```python
from build123d import *

# Parameters (mm, degrees)
SKETCH1_R                                       = 2.5
BOSS_EXTRUDE1_DEPTH                             = 35
SKETCH2_W                                       = 19.147849822
SKETCH2_H                                       = 14
CUT_EXTRUDE1_DEPTH                              = 11.980294351
CUT_EXTRUDE1_DEPTH_BACK                         = 1
CSK_FOR_M5_FLAT_HEAD_MACHINE_SCREW1_D           = 5.5
CSK_FOR_M5_FLAT_HEAD_MACHINE_SCREW1_DEPTH       = 13.347633298
CSK_FOR_M5_FLAT_HEAD_MACHINE_SCREW1_CSINK_D     = 10.4
CSK_FOR_M5_FLAT_HEAD_MACHINE_SCREW1_CSINK_ANGLE = 90
CSK_FOR_M5_FLAT_HEAD_MACHINE_SCREW1_TIP         = 1.652366702
CUT_EXTRUDE2_START                              = -14
SKETCH6_R                                       = 5.25
CUT_EXTRUDE2_DEPTH                              = 14
CUT_EXTRUDE3_START                              = -42
SKETCH6_2_R                                     = 5.25
CUT_EXTRUDE3_DEPTH                              = 14


with BuildPart() as part:
    # Sketch1 → Boss-Extrude1 (new body, symmetric)
    with BuildSketch(Plane(origin=(0, 0, 0), x_dir=(1, 0, 0), z_dir=(0, 1, 0))):
        with BuildLine():
            Line((0, 0), (28, 0))
            Line((28, 0), (28, -1.5))
            ThreePointArc((28, -1.5), (34.920820135, -7.683011565), (25.645751311, -8))
            Line((25.645751311, -8), (2.645751311, -8))
            Line((2.645751311, -8), (0, -5))
            Line((0, -5), (0, 0))
        make_face()
        with Locations((30.219676222, -5.980294351)):
            Circle(SKETCH1_R, mode=Mode.SUBTRACT)
    extrude(amount=BOSS_EXTRUDE1_DEPTH, both=True)

    # Sketch2 → Cut-Extrude1 (cut, two sides)
    with BuildSketch(Plane.XY) as cut_extrude1_sk:
        with Locations((35.219676222, 14)):
            Rectangle(SKETCH2_W, SKETCH2_H)
        with Locations((35.219676222, -14)):
            Rectangle(SKETCH2_W, SKETCH2_H)
    extrude(amount=CUT_EXTRUDE1_DEPTH, mode=Mode.SUBTRACT)
    extrude(cut_extrude1_sk.sketch, amount=-CUT_EXTRUDE1_DEPTH_BACK, mode=Mode.SUBTRACT)

    # CSK for M5 Flat Head Machine Screw1
    with Locations(Plane.XY.offset(8)):
        with Locations((12.432713767, 18), (12.432713767, -18)):
            CounterSinkHole(CSK_FOR_M5_FLAT_HEAD_MACHINE_SCREW1_D / 2, CSK_FOR_M5_FLAT_HEAD_MACHINE_SCREW1_CSINK_D / 2, depth=CSK_FOR_M5_FLAT_HEAD_MACHINE_SCREW1_DEPTH, counter_sink_angle=CSK_FOR_M5_FLAT_HEAD_MACHINE_SCREW1_CSINK_ANGLE)
            with Locations((0, 0, -(CSK_FOR_M5_FLAT_HEAD_MACHINE_SCREW1_DEPTH + CSK_FOR_M5_FLAT_HEAD_MACHINE_SCREW1_TIP / 2))):  # 118° drill point
                Cone(0, CSK_FOR_M5_FLAT_HEAD_MACHINE_SCREW1_D / 2, CSK_FOR_M5_FLAT_HEAD_MACHINE_SCREW1_TIP, mode=Mode.SUBTRACT)

    # Sketch6 → Cut-Extrude2 (cut)
    with BuildSketch(Plane(origin=(0, 35, 0), x_dir=(1, 0, 0), z_dir=(0, 1, 0)).offset(CUT_EXTRUDE2_START)):
        with Locations((30.219676222, -5.980294351)):
            Circle(SKETCH6_R)
    extrude(amount=-CUT_EXTRUDE2_DEPTH, mode=Mode.SUBTRACT)

    # Sketch6<2> → Cut-Extrude3 (cut)
    with BuildSketch(Plane(origin=(0, 35, 0), x_dir=(1, 0, 0), z_dir=(0, 1, 0)).offset(CUT_EXTRUDE3_START)):
        with Locations((30.219676222, -5.980294351)):
            Circle(SKETCH6_2_R)
    extrude(amount=-CUT_EXTRUDE3_DEPTH, mode=Mode.SUBTRACT)


solid = part.part
```
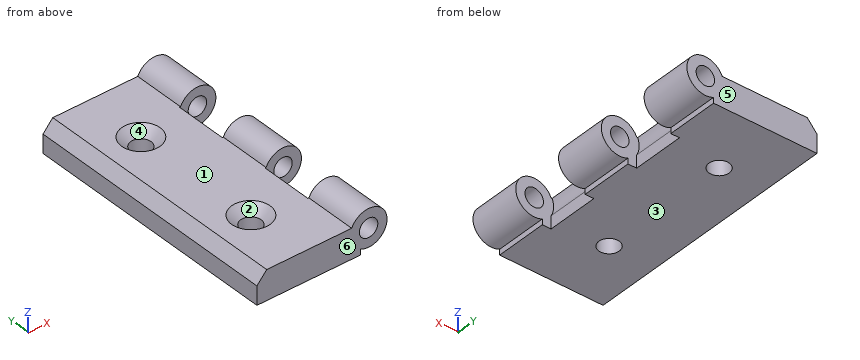
Design review of the part built by this model. Coordinates are the model's own, in mm. Face numbers are marked on the shaded views. A direction names the side the tool comes from. Round coordinates to 2 decimals unless told otherwise and drop trailing zeros. Write each loop counter-clockwise with the first axis right and the second up, starting at its lowest first coordinate (ties: lowest second). Pieces come first, ordered by that corner, then holes.
Item 1: We need section B-B on z = 2.25. Write out the cut boundary in (x, y).
Item 2: We need section D-D on x = 14.5. State how many separate pieces and enclosed holes the cut face has, and give its area (3 significant figures).
Item 3: The part is to be moulded in two halves that separate along Y. For the marked faces 3, 4, 5 and 6, say which applies: +Y half, -Y half, draft (parallel to the pull), parting line (faces both ways), or undercut.
Item 4: Clearance check with flat-ended pins moving along their axes: pin 1 Ø1 at (x, y) = (18, 22) entering from +Z; pin 2 Ø0.8 at (y, z) = (29.5, 0.5) entering from +X; pin 3 Ø1.5 at (y, z) = (-9.5, 6.5) entering from +X. State where each tip first meets the part, or that it passes through.
Item 5: We need section C-C on x = 33.5. Write out the cut boundary in (y, z).
Item 6: For probe 1 along Y at (x, z) = (12.5, 2.5); probe 2 along Y at (x, z) = (32, 8.75); probe 3 along X at (y, z) = (-2, 6.5), list the stretches that pass through material, from the lowest coordinate up.
Item 7: We need section A-A on y = -18. Write out the cut boundary in (x, z).
Item 8: For the marked faces 1 and 2, list the 3-axis set-ups (+Z, -Z, +X, -X, +Y, -Y) from which the entire face can be reached by the end or side of a thin tool; tool diameter is ignored.
Returned:
1. outline: (0, -35) - (33.55, -35) - (33.55, -21) - (25.65, -21) - (25.65, -7) - (33.55, -7) - (33.55, 7) - (25.65, 7) - (25.65, 21) - (33.55, 21) - (33.55, 35) - (0, 35) - close; hole circle Ø5.5 at (12.43, -18); hole circle Ø5.5 at (12.43, 18)
2. separate pieces: 3
2. enclosed holes: 0
2. area: 487 mm2
3. face 3: draft
3. face 4: undercut
3. face 5: +Y half
3. face 6: -Y half
4. pin 1: stops at z = 8
4. pin 2: stops at x = 28
4. pin 3: stops at x = 25.13
5. outline: (-35, 2.21) - (-21, 2.21) - (-21, 9.75) - (-35, 9.75) - close; (-7, 2.21) - (7, 2.21) - (7, 9.75) - (-7, 9.75) - close; (21, 2.21) - (35, 2.21) - (35, 9.75) - (21, 9.75) - close
6. probe 1: y = -35 to -20.75, -15.25 to 15.25, 20.75 to 35
6. probe 2: y = -35 to -21, -7 to 7, 21 to 35
6. probe 3: x = 1.32 to 27.77, 32.67 to 35.19
7. outline: (0, 0) - (9.68, 0) - (9.68, 5.55) - (7.23, 8) - (2.65, 8) - (0, 5) - close; (15.18, 0) - (25.65, 0) - (25.65, 3.4) arc R5.25 cw to (25.37, 8) - (17.63, 8) - (15.18, 5.55) - close
8. face 1: +Z, -X, +Y, -Y
8. face 2: +Z
